Part print with two shaded views. Sizes in mm from the minimum x, y, z corner. A direction names the side the tool comes from. Give positions to 0.01 mm unless a question says otherwise; leave off trailing zeros. Loops run counter-clockwise (first coordinate to the right, second up) from the corner with the lowest first, then second, coordinate; pieces in that order, holes last. Notation, with made-up numbers: M 8,32 L 43,32 A38 cw 43,70 Z; hole C 44,34 d6. An arc over 180 degrees is marked long. Answer in a Markdown table with one row per item.
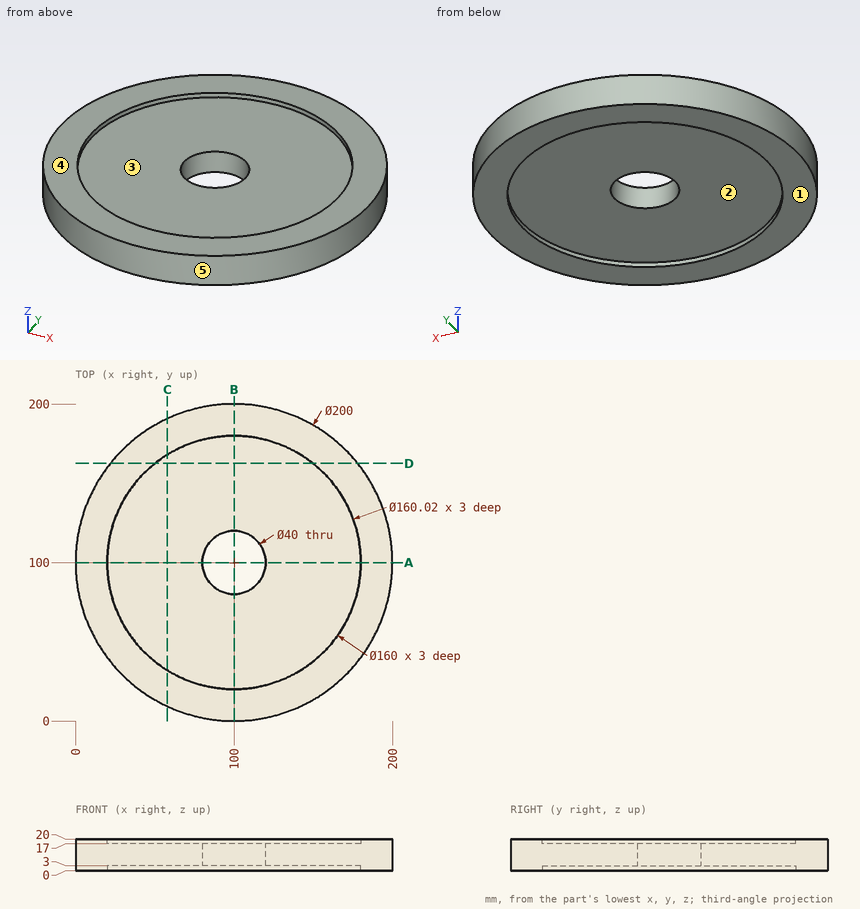
Q1. Probe probe 1 along Y at (x, z) = (100, 19.3); probe 2 along Y at (x, z) = (100, 13); probe 3 along Z at (x, y) = (77.5, 115). List the from-to ranges inside material, lowest first.
Reported:
| item | result |
|---|---|
| probe 1 | 0 to 20, 180 to 200 |
| probe 2 | 0 to 80, 120 to 200 |
| probe 3 | 3 to 17 |
Q2. Drop flat-ended pins along their axis: pin 1 (1.5 mm diameter, centred on x = 120, y = 51, fed in from +Z); pin 2 (10 mm diameter, centred on y = 64.5, z = 16.5, fed in from -X) (1 decimal); pin 3 (5 mm diameter, centred on y = 168, z = 14, fed in from +X). Give the stop position or say it passes through.
Reported:
| item | result |
|---|---|
| pin 1 | z = 17 |
| pin 2 | x = 4.8 |
| pin 3 | x = 175.56 |
Q3. 3-axis set-ups, long thin cutter, end or side, ignore diameter. For the marked faces 1 and 2: which of +Z, -Z, +X, -X, +Y, -Y reach the whole face in a straight line?
Reported:
| item | result |
|---|---|
| face 1 | -Z, +X, -X, +Y, -Y |
| face 2 | -Z |
Q4. Saw through at A-A (y = 100). Give the cut face in (x, z).
Reported:
| item | result |
|---|---|
| outline | M 0,0 L 19.99,0 L 19.99,3 L 80,3 L 80,17 L 20,17 L 20,20 L 0,20 Z; M 120,3 L 180.01,3 L 180.01,0 L 200,0 L 200,20 L 180,20 L 180,17 L 120,17 Z |
Q5. Saw through at D-D (y = 162.5). Give the cut face in (x, z), and give its area (3 significant figures).
Reported:
| item | result |
|---|---|
| outline | M 21.94,0 L 50.05,0 L 50.05,3 L 149.95,3 L 149.95,0 L 178.06,0 L 178.06,20 L 149.94,20 L 149.94,17 L 50.06,17 L 50.06,20 L 21.94,20 Z |
| area | 2,520 mm² |
Q6. Saw through at C-C (x = 58). Give the cut face in (y, z).
Reported:
| item | result |
|---|---|
| outline | M 9.25,0 L 31.9,0 L 31.9,3 L 168.1,3 L 168.1,0 L 190.75,0 L 190.75,20 L 168.09,20 L 168.09,17 L 31.91,17 L 31.91,20 L 9.25,20 Z |
Q7. Mould opens along Y. For the marked faces 3, 4 and 5 say: released by +Y, released by -Y, zero draft, split by the parting line, or undercut.
Reported:
| item | result |
|---|---|
| face 3 | undercut |
| face 4 | zero draft |
| face 5 | split by the parting line |
